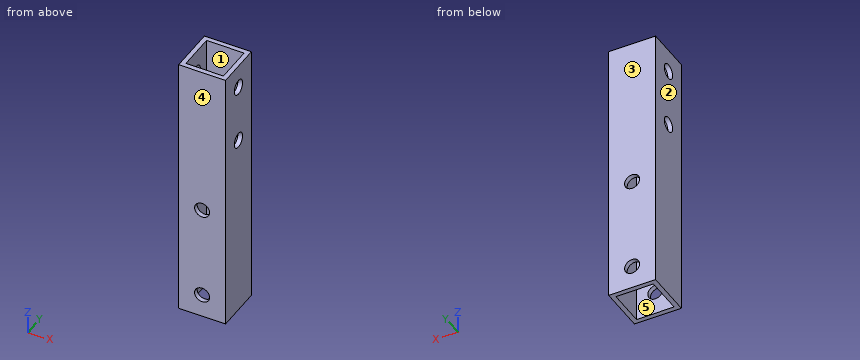
from build123d import *

# Parameters (mm, degrees)
SKETCH_1_W          = 10
SKETCH_1_H          = 10
SKETCH_1_W_2        = 8
SKETCH_1_H_2        = 8
EXTRUDE_1_DEPTH     = 57.5
SKETCH_2_R          = 1.6
CUT_EXTRUDE_1_DEPTH = 59.576872569
CUT_EXTRUDE_2_DEPTH = 10


with BuildPart() as part:
    # ｽｹｯﾁ1 → 押し出し-薄板1 (new body)
    with BuildSketch(Plane.XY):
        Rectangle(SKETCH_1_W, SKETCH_1_H)
        Rectangle(SKETCH_1_W_2, SKETCH_1_H_2, mode=Mode.SUBTRACT)
    extrude(amount=EXTRUDE_1_DEPTH)

    # ｽｹｯﾁ2 → ｶｯﾄ - 押し出し1 (cut, through all)
    with BuildSketch(Plane(origin=(0, 5, 0), x_dir=(1, 0, 0), z_dir=(0, 1, 0))):
        with Locations(Location((0, -5, 0), (0, 0, 270))):
            Circle(SKETCH_2_R)
        with Locations(Location((0, -25, 0), (0, 0, 270))):
            Circle(SKETCH_2_R)
    extrude(amount=-CUT_EXTRUDE_1_DEPTH, mode=Mode.SUBTRACT)

    # ｽｹｯﾁ4 → ｶｯﾄ - 押し出し2 (cut)
    with BuildSketch(Plane(origin=(5, 0, 0), x_dir=(0, 0, -1), z_dir=(1, 0, 0))):
        with BuildLine():
            ThreePointArc((-38.4, 0), (-40, 1.6), (-41.6, 0))
            Line((-41.6, 0), (-38.4, 0))
        make_face()
        with BuildLine():
            Line((-38.4, 0), (-41.6, 0))
            ThreePointArc((-41.6, 0), (-40, -1.6), (-38.4, 0))
        make_face()
        with BuildLine():
            ThreePointArc((-50.9, 0), (-52.5, 1.6), (-54.1, 0))
            Line((-54.1, 0), (-50.9, 0))
        make_face()
        with BuildLine():
            Line((-50.9, 0), (-54.1, 0))
            ThreePointArc((-54.1, 0), (-52.5, -1.6), (-50.9, 0))
        make_face()
    extrude(amount=-CUT_EXTRUDE_2_DEPTH, mode=Mode.SUBTRACT)


solid = part.part
Source: CAD feature listing. Evaluate the final solid. Frame: model axes, mm. Face numbers are marked on the shaded views. A direction names the side the tool comes from. Coordinates: 2 decimals unless noted, no trailing zeros. Loops run counter-clockwise (first coordinate to the right, second up) from the corner with the lowest first, then second, coordinate; pieces in that order, holes last. Notation, with made-up numbers: (87.5, 34.5) - (110.5, 34.5) arc R29 cw to (110.5, 71.5) - close; hole circle Ø10 at (42, -40). An arc over 180 degrees is marked (long way). Return JSON: item names as keys, results as strings.
Q1. Material intervals for line 1 along X through (y, z) = (-3.75, 38.5); line 2 along Y through (x, z) = (-4.3, 40); line 3 along Z through (x, y) = (4.4, 0), sorted ascending.
Results:
{"line 1": "-5 to -4, 4 to 5", "line 2": "-5 to -1.6, 1.6 to 5", "line 3": "0 to 38.4, 41.6 to 50.9, 54.1 to 57.5"}
Q2. Section D-D, the plane y = 0. Return loops of the section in (x, z).
Results:
{"outline": "(-5, 0) - (-4, 0) - (-4, 38.4) - (-5, 38.4) - close; (-5, 41.6) - (-4, 41.6) - (-4, 50.9) - (-5, 50.9) - close; (-5, 54.1) - (-4, 54.1) - (-4, 57.5) - (-5, 57.5) - close; (4, 0) - (5, 0) - (5, 38.4) - (4, 38.4) - close; (4, 41.6) - (5, 41.6) - (5, 50.9) - (4, 50.9) - close; (4, 54.1) - (5, 54.1) - (5, 57.5) - (4, 57.5) - close"}
Q3. Access query for the marked faces 4 and 5. Directions: +Z, -Z, +X, -X, +Y, -Y. A direction counts if a zero-diameter tool reaches every point of the face in a straight line with its end or side. Return the directions, or none.
Results:
{"face 4": "+Z, -Z, +X, -X, -Y", "face 5": "+Z, -Z"}
Q4. Contact query for a flat-ended pin moving along its axis: P1, Ø1.9, axis at x = 0, z = 25, coming from the -Y side. Output: stop coordinate, or through.
Results:
{"P1": "through"}
Q5. Section A-A, the plane y = 3.25. Return loops of the section in (x, z), plus the area to 3 significant figures.
Results:
{"outline": "(-5, 0) - (-4, 0) - (-4, 57.5) - (-5, 57.5) - close; (4, 0) - (5, 0) - (5, 57.5) - (4, 57.5) - close", "area": "115 mm2"}
Q6. Section C-C, the plane z = 25. Return loops of the section in (x, y).
Results:
{"outline": "(-5, -5) - (-1.6, -5) - (-1.6, -4) - (-4, -4) - (-4, 4) - (-1.6, 4) - (-1.6, 5) - (-5, 5) - close; (1.6, -5) - (5, -5) - (5, 5) - (1.6, 5) - (1.6, 4) - (4, 4) - (4, -4) - (1.6, -4) - close"}
Q7. Mould query, pull axis Y, two halves, no side actions, for the marked faces 1, 2 and 3. Classes: released by +Y, released by -Y, zero draft, split by the parting line, or undercut.
Results:
{"face 1": "undercut", "face 2": "zero draft", "face 3": "released by +Y"}
